Design review of the part built by this model. Coordinates are the model's own, in mm. Coordinates: 2 decimals unless noted, no trailing zeros. Write each loop counter-clockwise with the first axis right and the second up, starting at its lowest first coordinate (ties: lowest second). Pieces come first, ordered by that corner, then holes. Notation, with made-up numbers: M 64,25.5 L 71,25.5 A13 cw 71,48.5 Z; hole C 4,60 d1. An arc over 180 degrees is marked long. One line per question, with ' | ' between items.
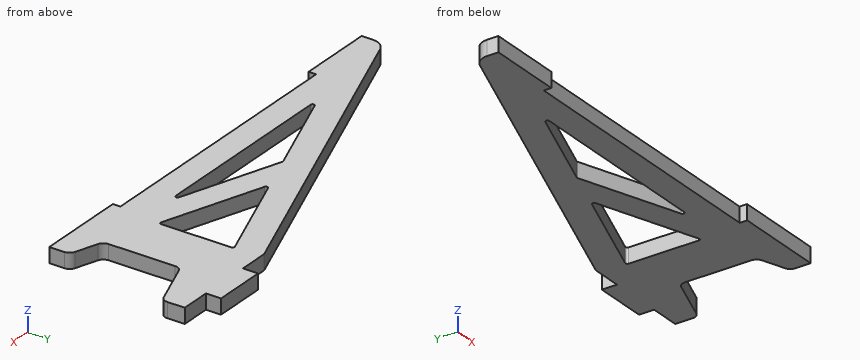
from build123d import *

# Parameters (mm, degrees)
BOSS_EXTRUDE1_DEPTH = 2


with BuildPart() as part:
    # Sketch1 → Boss-Extrude1 (new body)
    with BuildSketch(Plane.XY):
        with BuildLine():
            Line((1.315959713, 3.372369155), (47, 20))
            Line((47, 20), (51, 20))
            Line((51, 20), (51, 22))
            Line((51, 22), (58, 22))
            Line((58, 22), (58, 20))
            Line((58, 20), (62, 20))
            Line((62, 20), (62, 17.700207538))
            ThreePointArc((62, 17.700207538), (61.819152044, 17.126631102), (61.342020143, 16.760514917))
            Line((61.342020143, 16.760514917), (55.428944301, 14.608331318))
            ThreePointArc((55.428944301, 14.608331318), (54.9518124, 14.242215134), (54.770964445, 13.668638697))
            Line((54.770964445, 13.668638697), (54.770964445, 4.876414251))
            ThreePointArc((54.770964445, 4.876414251), (54.956848926, 4.295711295), (55.44539629, 3.930895675))
            Line((55.44539629, 3.930895675), (58.325568154, 2.939172971))
            ThreePointArc((58.325568154, 2.939172971), (58.814115518, 2.574357351), (59, 1.993654396))
            Line((59, 1.993654396), (59, 0))
            Line((59, 0), (47, 0))
            Line((47, 0), (47, 1))
            Line((47, 1), (10, 1))
            Line((10, 1), (10, 0))
            Line((10, 0), (0, 0))
            Line((0, 0), (0, 1.492983913))
            ThreePointArc((0, 1.492983913), (0.361695911, 2.640136786), (1.315959713, 3.372369155))
        make_face()
        with BuildLine():
            Line((15.979730818, 4.984923155), (28.367873469, 9.493838338))
            ThreePointArc((28.367873469, 9.493838338), (28.451196871, 9.508905664), (28.534770543, 9.495294827))
            Line((28.534770543, 9.495294827), (41.629611064, 4.986379644))
            ThreePointArc((41.629611064, 4.986379644), (41.794790425, 4.708738099), (41.548219025, 4.5))
            Line((41.548219025, 4.5), (16.065235854, 4.5))
            ThreePointArc((16.065235854, 4.5), (15.819033916, 4.706587956), (15.979730818, 4.984923155))
        make_face(mode=Mode.SUBTRACT)
        with BuildLine():
            Line((47.770964445, 16.198948904), (47.770964445, 6.92390155))
            ThreePointArc((47.770964445, 6.92390155), (47.666140184, 6.72037267), (47.439572406, 6.687521906))
            Line((47.439572406, 6.687521906), (34.344731886, 11.196437088))
            ThreePointArc((34.344731886, 11.196437088), (34.176133444, 11.430635098), (34.340618889, 11.667739888))
            Line((34.340618889, 11.667739888), (47.435459409, 16.433872059))
            ThreePointArc((47.435459409, 16.433872059), (47.664358554, 16.403736915), (47.770964445, 16.198948904))
        make_face(mode=Mode.SUBTRACT)
    extrude(amount=BOSS_EXTRUDE1_DEPTH)


solid = part.part
1. Take a section at A-A (z = 1.1). Count the separate pieces of the cut face and the enclosed holes in it, then the cut area to 3 significant figures.
Answer sheet:
separate pieces: 1 | enclosed holes: 2 | area: 575 mm^2
2. Take a section at B-B (x = 27.5). Write out the cut boundary in (y, z).
Answer sheet:
outline: M 1,0 L 4.5,0 L 4.5,2 L 1,2 Z; M 9.18,0 L 12.9,0 L 12.9,2 L 9.18,2 Z
3. Take a section at C-C (y = 15.25). Write out the cut boundary in (x, z), then the cut area to 3 significant figures.
Answer sheet:
outline: M 33.95,0 L 44.18,0 L 44.18,2 L 33.95,2 Z; M 47.77,0 L 57.19,0 L 57.19,2 L 47.77,2 Z | area: 39.3 mm^2
4. To check wall thickness, follow line 1 along X through (y, z) = (21, 0.65); line 2 along Y through (x, z) = (43, 0.8); line 3 along Y through (x, z) = (56, 0.35). State the ranges of each line that lie inside material, in increasing order. Write a range as [from, to].
Answer sheet:
line 1: [51, 58] | line 2: [1, 8.22], [14.82, 18.54] | line 3: [0, 3.74], [14.82, 22]
5. Insertion check: pin 1 Ø0.6 at (x, z) = (49, 1) entering from +Y; pin 2 Ø1 at (x, z) = (16.5, 1) entering from +Y; pin 3 Ø0.8 at (y, z) = (0.5, 1.5) entering from +X. Each pin has a flat end and moves straight along its axis. Give the tip position at first contact, or say it passes through.
Answer sheet:
pin 1: y = 20 | pin 2: y = 9.08 | pin 3: x = 59
6. Take a section at D-D (x = 7). Write out the cut boundary in (y, z), then the cut area to 3 significant figures.
Answer sheet:
outline: M 0,0 L 5.44,0 L 5.44,2 L 0,2 Z | area: 10.9 mm^2
